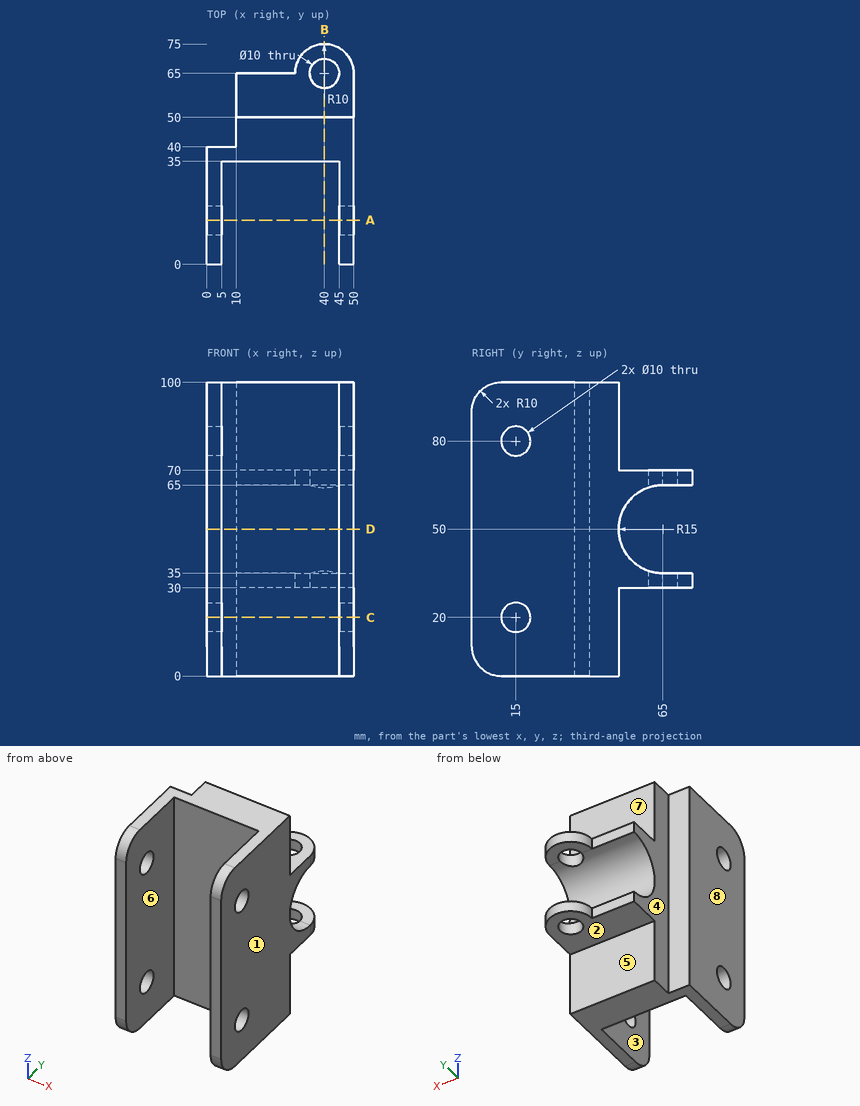
Design review of the part shown in the three views and the two pictorial views. Dimensions are in mm from the part's minimum x, y and z. A direction names the side the tool comes from. Round coordinates to 2 decimals unless told otherwise and drop trailing zeros. Write each loop counter-clockwise with the first axis right and the second up, starting at its lowest first coordinate (ties: lowest second). Pieces come first, ordered by that corner, then holes. Notation, with made-up numbers: (78, 1) - (94, 1) arc R22 ccw to (94, 18) - close; hole circle Ø1 at (-29.5, 19). An arc over 180 degrees is marked (long way). Return JSON: item names as keys, results as strings. Group by question number.
Item 1: For probe 1 along X at (y, z) = (34.5, 92); probe 2 along Y at (x, z) = (40, 66.6); probe 3 along Y at (x, z) = (12, 6.5), list the stretches that pass through material, from the lowest coordinate up. Write a range as [from, to].
Item 2: Machinability: for the marked faces 4, 5, 6, 7 and 8, which of the approach directions +Z, -Z, +X, -X, +Y, -Y give a long, thin tool a straight path to every point of the face, cutting with its end or side? Answer none if there is none.
Item 3: We need section A-A on y = 15. Write out the cut boundary in (x, z).
Item 4: The part is to be moulded in two halves that separate along X. For the marked faces 1, 2 and 3, say which applies: pulls with the +X half, pulls with the -X half, needs draft (parallel to the pull), parting line crosses it, or undercut.
Item 5: We need section C-C on z = 20. Write out the cut boundary in (x, y), and give its area (3 significant figures).
Item 6: Insertion check: P1, Ø10, axis at x = 26.5, z = 22, coming from the -Y side; P2, Ø11, axis at x = 38, y = 71, coming from the -Z side; P3, Ø3, axis at x = 39, y = 68.5, coming from the +Z side. Each pin has a flat end and moves straight along its axis. Give the tip position at first contact, or say it passes through.
Item 7: We need section B-B on x = 40. Write out the cut boundary in (y, z), and give its area (3 significant figures).
Item 8: We need section D-D on z = 50. Write out the cut boundary in (x, y).
Model answer:
{
 "1": {"probe 1": "x = [0, 5], [45, 50]", "probe 2": "y = [35, 60], [70, 75]", "probe 3": "y = [35, 50]"},
 "2": {"face 4": "+Z, -Z, -X, +Y", "face 5": "-Z, +X, -X, +Y", "face 6": "+Z, -Z, -Y", "face 7": "+Z, +X, -X, +Y", "face 8": "+Z, -Z, -X, +Y, -Y"},
 "3": {"outline": "(0, 0) - (5, 0) - (5, 15) - (0, 15) - close; (0, 25) - (5, 25) - (5, 75) - (0, 75) - close; (0, 85) - (5, 85) - (5, 100) - (0, 100) - close; (45, 0) - (50, 0) - (50, 15) - (45, 15) - close; (45, 25) - (50, 25) - (50, 75) - (45, 75) - close; (45, 85) - (50, 85) - (50, 100) - (45, 100) - close"},
 "4": {"face 1": "pulls with the +X half", "face 2": "needs draft", "face 3": "undercut"},
 "5": {"outline": "(0, 0) - (5, 0) - (5, 10) - (0, 10) - close; (0, 20) - (5, 20) - (5, 35) - (45, 35) - (45, 20) - (50, 20) - (50, 50) - (10, 50) - (10, 40) - (0, 40) - close; (45, 0) - (50, 0) - (50, 10) - (45, 10) - close", "area": "900 mm²"},
 "6": {"P1": "stops at y = 35", "P2": "stops at z = 30", "P3": "stops at z = 70"},
 "7": {"outline": "(35, 0) - (50, 0) - (50, 30) - (60, 30) - (60, 35.86) arc R15 cw to (60, 64.14) - (60, 70) - (50, 70) - (50, 100) - (35, 100) - close; (70, 30) - (75, 30) - (75, 35) - (70, 35) - close; (70, 65) - (75, 65) - (75, 70) - (70, 70) - close", "area": "1,740 mm²"},
 "8": {"outline": "(0, 0) - (5, 0) - (5, 35) - (45, 35) - (45, 0) - (50, 0) - (50, 50) - (10, 50) - (10, 40) - (0, 40) - close"}
}
